Verification items for the finished model (mm, model axes). A direction names the side the tool comes from. Give positions to 0.01 mm unless a question says otherwise; leave off trailing zeros. Loops run counter-clockwise (first coordinate to the right, second up) from the corner with the lowest first, then second, coordinate; pieces in that order, holes last. Notation, with made-up numbers: M -16.75,66.25 L -9.75,66.25 A24 ccw -9.75,100.25 Z; hole C 18.5,-26 d2. An arc over 180 degrees is marked long. Use a Markdown table: item, result.
from build123d import *

# Parameters (mm, degrees)
ESQUISSE1_R                         = 9.5
BOSS_EXTRU_1_DEPTH                  = 7
ESQUISSE2_W                         = 5.8
ESQUISSE2_H                         = 2.4
ENL_V_MAT_EXTRU_1_DEPTH             = 6
ENL_V_MAT_EXTRU_2_REACH             = 19.336
ESQUISSE3_R                         = 1.6
ENL_V_MAT_EXTRU_2_DIRECTION_2_REACH = 19.336
ESQUISSE7_R                         = 2.95
ENL_V_MAT_EXTRU_8_DEPTH             = 22.858865638
CHANFREIN1_SIZE                     = 2
ESQUISSE9_R                         = 3.9
BOSS_EXTRU_2_DEPTH                  = 7


with BuildPart() as part:
    # Esquisse1 → Boss.-Extru.1 (new body)
    with BuildSketch(Plane.XY):
        Circle(ESQUISSE1_R)
        with BuildLine():
            Line((-1.565247584, 2.2), (1.565247584, 2.2))
            ThreePointArc((1.565247584, 2.2), (0, -2.7), (-1.565247584, 2.2))
        make_face(mode=Mode.SUBTRACT)
    extrude(amount=BOSS_EXTRU_1_DEPTH)

    # Esquisse2 → Enlèv. mat.-Extru.1 (cut)
    with BuildSketch(Plane(origin=(0, 0, 0), x_dir=(-1, 0, 0), z_dir=(0, 0, -1))):
        with Locations((0, 4.4)):
            Rectangle(ESQUISSE2_W, ESQUISSE2_H)
    extrude(amount=-ENL_V_MAT_EXTRU_1_DEPTH, mode=Mode.SUBTRACT)

    # Esquisse3 → Enlèv. mat.-Extru.2 (cut, up to next)
    with BuildSketch(Plane(origin=(0, 3.2, 0), x_dir=(1, 0, 0), z_dir=(0, 1, 0)), mode=Mode.PRIVATE) as enl_v_mat_extru_2_sk1:
        with Locations(Location((0, -3, 0), (0, 0, 90))):
            Circle(ESQUISSE3_R)
    enl_v_mat_extru_2_tool1 = extrude(enl_v_mat_extru_2_sk1.sketch, amount=-ENL_V_MAT_EXTRU_2_REACH, mode=Mode.PRIVATE) & part.part
    add(enl_v_mat_extru_2_tool1.solids().sort_by_distance((0, 3.2, 3))[0], mode=Mode.SUBTRACT)

    # Esquisse3 → Enlèv. mat.-Extru.2 direction 2 (cut, up to next)
    with BuildSketch(Plane(origin=(0, 3.2, 0), x_dir=(1, 0, 0), z_dir=(0, 1, 0)), mode=Mode.PRIVATE) as enl_v_mat_extru_2_direction_2_sk1:
        with Locations(Location((0, -3, 0), (0, 0, 90))):
            Circle(ESQUISSE3_R)
    enl_v_mat_extru_2_direction_2_tool1 = extrude(enl_v_mat_extru_2_direction_2_sk1.sketch, amount=ENL_V_MAT_EXTRU_2_DIRECTION_2_REACH, mode=Mode.PRIVATE) & part.part
    add(enl_v_mat_extru_2_direction_2_tool1.solids().sort_by_distance((0, 3.2, 3))[0], mode=Mode.SUBTRACT)

    # Esquisse7 → Enlèv. mat.-Extru.8 (cut, through all)
    with BuildSketch(Plane(origin=(0, 8.9, 0), x_dir=(1, 0, 0), z_dir=(0, 1, 0))):
        with Locations(Location((0, -3, 0), (0, 0, 90))):
            Circle(ESQUISSE7_R)
    extrude(amount=ENL_V_MAT_EXTRU_8_DEPTH, mode=Mode.SUBTRACT)

    # Chanfrein1
    # the kernel refuses this chamfer: 2 mm, written as the material it takes off along each edge
    with BuildSketch(Plane(origin=(0, 8.9, 3), x_dir=(0, 0, -1), z_dir=(-1, 0, 0))) as chanfrein1_piece_1_section:
        Polygon((1.6 + CHANFREIN1_SIZE, 0), (1.6, CHANFREIN1_SIZE), (1.6, 0), align=None)
    chanfrein1_piece_1 = revolve(axis=Axis((0, 8.9, 3), (0, -1, 0)), mode=Mode.PRIVATE)
    chanfrein1_piece_1 = chanfrein1_piece_1 & Plane(origin=(0, 7.567667742, 3), x_dir=(0, 0, -1), z_dir=(0, -1, 0)) * Cylinder(2.95, 15, mode=Mode.PRIVATE)
    add(chanfrein1_piece_1, mode=Mode.SUBTRACT)

    # Esquisse9 → Boss.-Extru.2 (add)
    with BuildSketch(Plane.XY.offset(7)):
        with Locations((0, -1)):
            Circle(ESQUISSE9_R)
        with BuildLine():
            Line((-1.565247584, 2.2), (1.565247584, 2.2))
            ThreePointArc((1.565247584, 2.2), (0, -2.7), (-1.565247584, 2.2))
        make_face(mode=Mode.SUBTRACT)
    extrude(amount=BOSS_EXTRU_2_DEPTH)


solid = part.part
(1) Cross-section at A-A on x = 0. Record the cut outline in (y, z), then the cut area to 3 significant figures.
Results below:
| item | result |
|---|---|
| outline | M -9.5,0 L -2.7,0 L -2.7,14 L -4.9,14 L -4.9,7 L -9.5,7 Z; M 2.2,0 L 3.2,0 L 3.2,1.4 L 2.2,1.4 Z; M 2.2,4.6 L 3.2,4.6 L 3.2,6 L 5.6,6 L 5.6,4.6 L 6.9,4.6 L 8.25,5.95 L 9.5,5.95 L 9.5,7 L 2.9,7 L 2.9,14 L 2.2,14 Z; M 5.6,0 L 9.5,0 L 9.5,0.05 L 8.25,0.05 L 6.9,1.4 L 5.6,1.4 Z |
| area | 83.7 mm^2 |
(2) Cross-section at C-C on z = 13. Record the cut outline in (x, y).
Results below:
| item | result |
|---|---|
| outline | C 0,-1 d7.8; hole M -1.57,2.2 A2.7 ccw long 1.57,2.2 Z |
(3) Set-up check for faces 4 (the flat face through (-2.2, -2, 0)), 5 (the cylindrical face through (-3.095, -3.373, 10.451)), 6 (the cylindrical face through (0.97, 2.69, 4.27)), 7 (the flat face through (0, 4, 6)), 8 (the flat face through (0, 2.2, 1)): record each of +Z, -Z, +X, -X, +Y, -Y from which the full face is reachable in a straight line by a thin tool's end or side.
Results below:
| item | result |
|---|---|
| face 4 | -Z, +X, -X, +Y, -Y |
| face 5 | +Z |
| face 6 | +Y |
| face 7 | -Z |
| face 8 | +Z, -Z |
(4) Cross-section at D-D on z = 3. Record the cut outline in (x, y).
Results below:
| item | result |
|---|---|
| outline | M -2.95,8.25 L -2.95,9.03 A9.5 ccw long 2.95,9.03 L 2.95,8.25 L 1.6,6.9 L 1.6,5.6 L 2.9,5.6 L 2.9,3.2 L 1.6,3.2 L 1.6,2.17 A2.7 cw long -1.6,2.17 L -1.6,3.2 L -2.9,3.2 L -2.9,5.6 L -1.6,5.6 L -1.6,6.9 Z |
(5) Gauge pin test, flat ends, axial feed: P1, Ø1.9, axis at x = 0, y = 4.5, coming from the -Z side; P2, Ø2.5, axis at x = 0, z = 3, coming from the +Y side; P3, Ø3, axis at x = 0, y = 0, coming from the +Z side; P4, Ø0.7, axis at y = 4, z = 2, coming from the +X side. Record the tip position at first contact, or that the pin passes through.
Results below:
| item | result |
|---|---|
| P1 | z = 6 |
| P2 | y = -2.39 |
| P3 | through |
| P4 | x = 8.77 |
(6) Cross-section at B-B on y = 1.25. Record the cut outline in (x, z), then the cut area to 3 significant figures.
Results below:
| item | result |
|---|---|
| outline | M -9.42,0 L -2.39,0 L -2.39,14 L -3.19,14 L -3.19,7 L -9.42,7 Z; M 2.39,0 L 9.42,0 L 9.42,7 L 3.19,7 L 3.19,14 L 2.39,14 Z |
| area | 109 mm^2 |
(7) Draft check along Z on faces 1 (the cylindrical face through (-0.886, 8.731, 0.186)), 2 (the flat face through (1.3, 3.2, 1.6)), 3 (the flat face through (4, 0, 7)). Enter one of: +Z half, -Z half, draft (parallel to the pull), parting line (faces both ways), or undercut.
Results below:
| item | result |
|---|---|
| face 1 | undercut |
| face 2 | draft |
| face 3 | +Z half |
(8) Material ranges on line 1 (Y direction, x = 1.5, z = 1.5) (3 decimals); line 2 (Z direction, x = -2.25, y = -6); line 3 (Y direction, x = -2, z = 1.75), recorded low to high.
Results below:
| item | result |
|---|---|
| line 1 | -9.381 to -2.245, 2.2 to 3.2, 5.6 to 7.421 |
| line 2 | 0 to 7 |
| line 3 | -9.29 to -1.81, 1.81 to 3.2, 5.6 to 7.66 |
